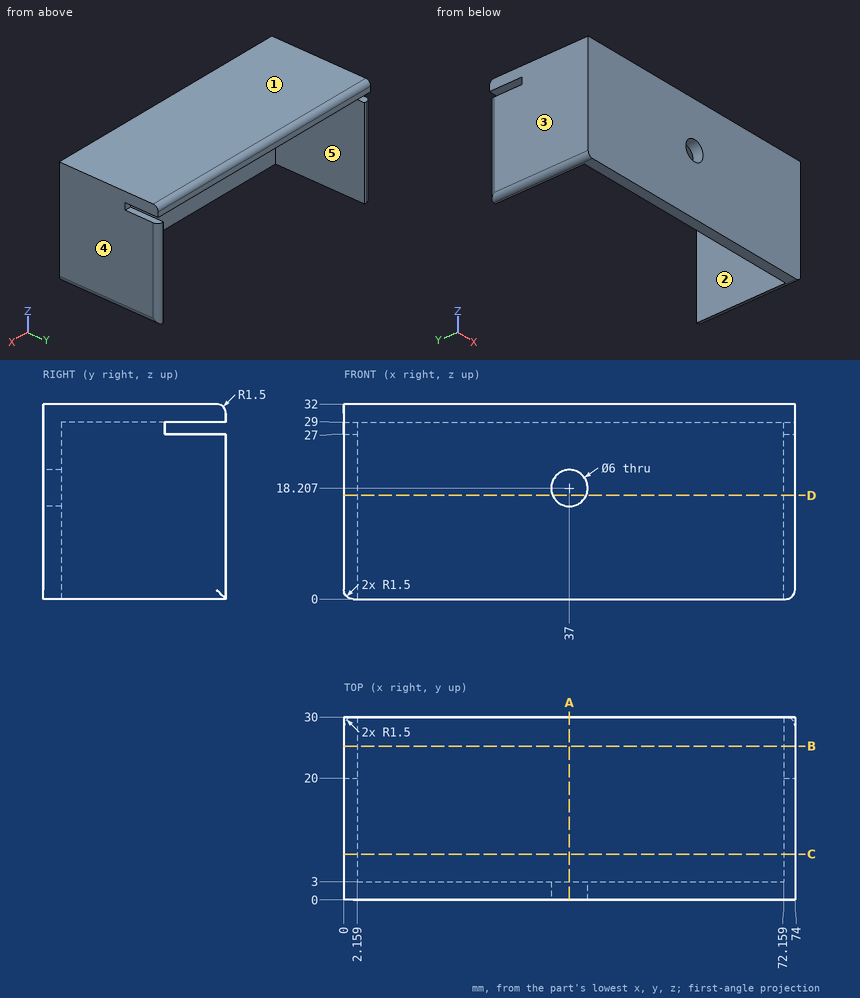
Input: dimensioned drawing with shaded views. Units: mm. Origin: part minimum x, y, z. A direction names the side the tool comes from. Coordinates: 2 decimals unless noted, no trailing zeros. Order: outer loops, then holes, each group sorted by start corner. A loop starts at its lowest first (then second) coordinate and runs counter-clockwise, first axis right, second up. Notation, with made-up numbers: (55, -3.5) - (61, -3.5) arc R16 ccw to (61, 6.5) - close; hole circle Ø7 at (25, 59.25). An arc over 180 degrees is marked (long way). Return JSON: item names as keys, results as strings. Group by question number.
1. Set-up query: the marked faces 1 and 2. Return all of +Z, -Z, +X, -X, +Y, -Y with unobstructed straight access to the full face (end or side cutting, diameter ignored); none if empty.
2. Pull-direction query (X, two-part tool) for the marked faces 3, 4 and 5; classes: pulls with the +X half, pulls with the -X half, needs draft (parallel to the pull), parting line crosses it, or undercut.
3. Cut plane D-D (z = 17). Output: boundary loops of the cut face in (x, y).
4. Cut plane C-C (y = 7.5). Output: boundary loops of the cut face in (x, z), plus the area to 3 significant figures.
5. Cut plane B-B (y = 25.25). Output: boundary loops of the cut face in (x, z).
6. Material intervals for line 1 along X through (y, z) = (6.5, 21.5); line 2 along Z through (x, y) = (37, 1.1); line 3 along Z through (x, y) = (4, 9.25), sorted ascending. Write a range as [from, to].
7. Pin query (flat end, axial travel): pin 1 (8 mm diameter, centred on y = 22.5, z = 21, fed in from -X); pin 2 (8 mm diameter, centred on x = 38.5, y = 27, fed in from -Z); pin 3 (5 mm diameter, centred on x = 37, z = 18.21, fed in from +Y); pin 4 (0.9 mm diameter, centred on x = 73, z = 28.5, fed in from +Y). Return the tip coordinate at first contact, or that it passes through.
8. Cut plane A-A (x = 37). Output: boundary loops of the cut face in (y, z).
Resolved:
{
 "1": {"face 1": "+Z, +X, -X, +Y, -Y", "face 2": "-Z, +Y"},
 "2": {"face 3": "pulls with the -X half", "face 4": "pulls with the +X half", "face 5": "undercut"},
 "3": {"outline": "(0, 0) - (34.25, 0) - (34.25, 3) - (2.16, 3) - (2.16, 30) - (1.5, 30) arc R1.5 ccw to (0, 28.5) - close; (39.75, 0) - (74, 0) - (74, 28.5) arc R1.5 ccw to (72.5, 30) - (72.16, 30) - (72.16, 3) - (39.75, 3) - close"},
 "4": {"outline": "(0, 1.5) arc R1.5 ccw to (1.5, 0) - (2.16, 0) - (2.16, 29) - (72.16, 29) - (72.16, 0) - (72.5, 0) arc R1.5 ccw to (74, 1.5) - (74, 32) - (0, 32) - close", "area": "337 mm²"},
 "5": {"outline": "(0, 1.5) arc R1.5 ccw to (1.5, 0) - (2.16, 0) - (2.16, 27) - (0, 27) - close; (0, 29) - (74, 29) - (74, 32) - (0, 32) - close; (72.16, 0) - (72.5, 0) arc R1.5 ccw to (74, 1.5) - (74, 27) - (72.16, 27) - close"},
 "6": {"line 1": "x = [0, 2.16], [72.16, 74]", "line 2": "z = [0, 15.21], [21.21, 32]", "line 3": "z = [29, 32]"},
 "7": {"pin 1": "stops at x = 0", "pin 2": "stops at z = 29", "pin 3": "passes through", "pin 4": "stops at y = 20"},
 "8": {"outline": "(0, 0) - (3, 0) - (3, 15.21) - (0, 15.21) - close; (0, 21.21) - (3, 21.21) - (3, 29) - (30, 29) - (30, 30.5) arc R1.5 ccw to (28.5, 32) - (0, 32) - close"}
}
